Design review of the part built by this model. Coordinates are the model's own, in mm. Face numbers are marked on the shaded views. A direction names the side the tool comes from. Round coordinates to 2 decimals unless told otherwise and drop trailing zeros. Write each loop counter-clockwise with the first axis right and the second up, starting at its lowest first coordinate (ties: lowest second). Pieces come first, ordered by that corner, then holes. Notation, with made-up numbers: M 75,12.5 L 91,12.5 A27 ccw 91,38.5 Z; hole C 19,50.5 d1. An arc over 180 degrees is marked long. One line per question, with ' | ' between items. Start each with the question number.
Item 1: Add section B-B, the plane x = -88. State the section outline as (y, z) points.
Item 2: Machinability: for the marked faces 5, 6 and 7, which of the approach directions +Z, -Z, +X, -X, +Y, -Y give a long, thin tool a straight path to every point of the face, cutting with its end or side? Answer none if there is none.
Item 3: Add section A-A, the plane y = 12. State the section outline as (x, z) points.
Item 4: For L1, parallel to Y at x = -88, z = 9.25; L2, parallel to Y at x = -88, z = 12.05; L3, parallel to X at y = 12, z = 12, list the stretches that pass through material, from the lowest coordinate up.
Item 5: Draft analysis for pull direction Y (two halves, no side actions). For the marked faces 1, 2, 3 and 4, state which applies: released by +Y, released by -Y, zero draft, split by the parting line, or undercut.
Item 6: Insertion check: pin 1 Ø3 at (x, y) = (-86.5, 16.5) entering from -Z; pin 2 Ø4 at (x, z) = (-84, 7) entering from -Y. Each pin has a flat end and moves straight along its axis. Give the tip position at first contact, or say it passes through.
Item 7: Add section C-C, the plane z = 11.5. State the section outline as (x, y) points, and give its area (3 significant figures).
```python
from build123d import *

# Parameters (mm, degrees)
SKETCH073_W             = 2.501097
SKETCH073_H             = 5.003426
POCKET017_DEPTH         = 0.5
POLARPATTERN_COUNT      = 8
BODY016_PLACEMENT_ANGLE = 22.5


with BuildPart() as part:
    # Sketch072 → Revolution005 (revolve)
    with BuildSketch(Plane.XZ):
        Polygon((5.321734, 8.4), (5.321734, 7.168998), (6.315841, 7.168998), (6.315841, 4.11532), (6.434004, 4.11532), (6.633604, 2.430329), (6.336122, 1.240818), (6.621345, 0.904052), (6.621345, 0.689515), (6.725548, 0.193016), (8, 0.193016), (8, 8.4), align=None)
    revolve(axis=Axis((0, 0, 0), (0, 0, 1)))

    # Sketch073 → Pocket017 (cut, symmetric)
    with BuildSketch(Plane.XZ):
        with Locations((7.439441, 2.501713)):
            Rectangle(SKETCH073_W, SKETCH073_H)
    pocket017 = extrude(amount=POCKET017_DEPTH, both=True, mode=Mode.SUBTRACT)

    # PolarPattern: Pocket017 ×8 about axis
    polarpattern_axis = Axis((0, 0, 0), (0, 0, 1))
    for i in range(1, POLARPATTERN_COUNT):
        add(pocket017.rotate(polarpattern_axis, i * 360 / POLARPATTERN_COUNT), mode=Mode.SUBTRACT)


with BuildPart() as part_1:
    # Body016 placement: moved
    add(part.part.moved(Location((-88, 12, 4))).rotate(Axis((-88, 12, 4), (0, 0, -1)), BODY016_PLACEMENT_ANGLE))


solid = part_1.part
```
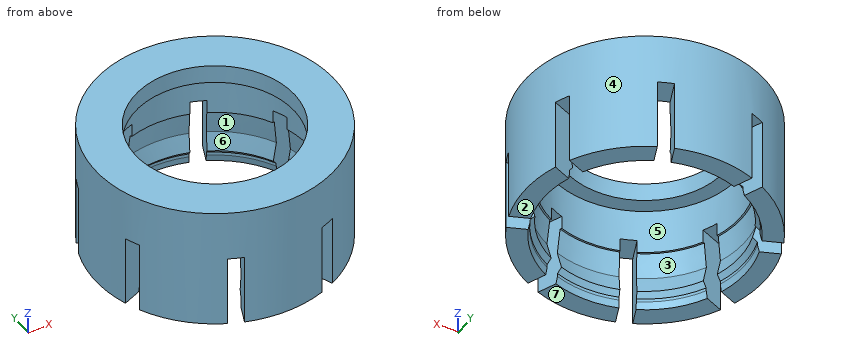
Computed values:
1) outline: M 4,4.19 L 5.27,4.19 L 5.38,4.69 L 5.38,4.9 L 5.66,5.24 L 5.37,6.43 L 5.57,8.12 L 5.68,8.12 L 5.68,11.17 L 6.68,11.17 L 6.68,12.4 L 4,12.4 Z; M 17.32,11.17 L 18.32,11.17 L 18.32,8.12 L 18.43,8.12 L 18.63,6.43 L 18.34,5.24 L 18.62,4.9 L 18.62,4.69 L 18.73,4.19 L 20,4.19 L 20,12.4 L 17.32,12.4 Z
2) face 5: -Z | face 6: none | face 7: -Z, +X, -X, +Y, -Y
3) outline: M -96,4.19 L -94.73,4.19 L -94.62,4.69 L -94.62,4.9 L -94.34,5.24 L -94.63,6.43 L -94.43,8.12 L -94.32,8.12 L -94.32,11.17 L -93.32,11.17 L -93.32,12.4 L -96,12.4 Z; M -82.68,11.17 L -81.68,11.17 L -81.68,8.12 L -81.57,8.12 L -81.37,6.43 L -81.66,5.24 L -81.38,4.9 L -81.38,4.69 L -81.27,4.19 L -80,4.19 L -80,12.4 L -82.68,12.4 Z
4) L1: y = 4 to 5.68, 18.32 to 20 | L2: y = 4 to 6.68, 17.32 to 20 | L3: x = -96 to -93.32, -82.68 to -80
5) face 1: undercut | face 2: zero draft | face 3: undercut | face 4: split by the parting line
6) pin 1: stops at z = 11.17 | pin 2: stops at y = 4.25
7) outline: C -88,12 d16; hole C -88,12 d10.64 | area: 112 mm^2
